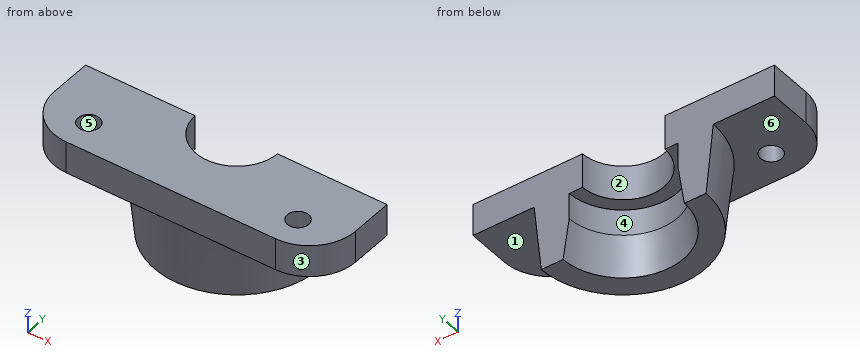
from build123d import *
from OCP.BRepAlgoAPI import BRepAlgoAPI_Cut
from OCP.TopTools import TopTools_ListOfShape

# Parameters (mm, degrees)
BOSS_EXTRUDE2_DEPTH      = 22.67949
BOSS_EXTRUDE2_DEPTH_BACK = 22.67949
SKETCH5_R                = 1.6
CUT_EXTRUDE1_DEPTH       = 29.214793281


with BuildPart() as part:
    # Sketch3 → Boss-Extrude2 (new, two sides: drawn at the far end of the back side and taken through both)
    with BuildSketch(Plane(origin=(0, 0, 0), x_dir=(0, 0, -1), z_dir=(1, 0, 0)).offset(-BOSS_EXTRUDE2_DEPTH_BACK)):
        Polygon((4.8, -13.329489609), (0, -13.329489609), (0, 0), (15, 0), (15, -12.25742641), align=None)
    extrude(amount=BOSS_EXTRUDE2_DEPTH + BOSS_EXTRUDE2_DEPTH_BACK)

    # Sketch2 → Cut-Revolve1 (revolve, cut)
    with BuildSketch(Plane(origin=(0, 0, 0), x_dir=(0, 0, -1), z_dir=(1, 0, 0))):
        Polygon((15, 0.15), (0, 0.15), (0, -6.05), (5.2, -6.05), (5.2, -8.05), (9.121020847, -8.05), (15, -8.981138823), align=None)
    revolve(axis=Axis((0, 0.15, -15), (0, 0, 1)), mode=Mode.SUBTRACT)

    # Sketch4 → Cut-Revolve2 (revolve, cut)
    with BuildSketch(Plane(origin=(0, 0.15, -14), x_dir=(0, 0, -1), z_dir=(1, 0, 0))):
        Polygon((1, 12.40742641), (-9.2, 13.479489609), (-9.2, 37.679985647), (1, 37.679985647), align=None)
    revolve(axis=Axis((0, 0.15, -14), (0, 0, 1)), mode=Mode.SUBTRACT)


with BuildPart() as cut_extrude1_tool:
    # Sketch5 → Cut-Extrude1 (new, through all)
    with BuildSketch(Plane(origin=(0, 0, -4.8), x_dir=(-1, 0, 0), z_dir=(0, 0, -1))):
        with Locations(Location((-15.748733562, -8.729489609, 0), (0, 0, 90))):
            Circle(SKETCH5_R)
        with Locations(Location((15.748733562, -8.729489609, 0), (0, 0, 270))):
            Circle(SKETCH5_R)
        with BuildLine():
            Line((-22.679489609, -13.329489609), (-22.679489609, -6.398733562))
            ThreePointArc((-22.679489609, -6.398733562), (-20.649518162, -11.299518162), (-15.748733562, -13.329489609))
            Line((-15.748733562, -13.329489609), (-22.679489609, -13.329489609))
        make_face()
        with BuildLine():
            Line((22.679489609, -13.329489609), (22.679489609, -6.398733562))
            ThreePointArc((22.679489609, -6.398733562), (20.649518162, -11.299518162), (15.748733562, -13.329489609))
            Line((15.748733562, -13.329489609), (22.679489609, -13.329489609))
        make_face()
    extrude(amount=-CUT_EXTRUDE1_DEPTH)


with BuildPart() as part_1:
    add(part.part)

    # Cut-Extrude1: cut by cut_extrude1_tool, with a tolerance
    cut_extrude1_stock = TopTools_ListOfShape()
    cut_extrude1_stock.Append(part_1.part.wrapped)
    cut_extrude1_tools = TopTools_ListOfShape()
    cut_extrude1_tools.Append(cut_extrude1_tool.part.wrapped)
    cut_extrude1_cut = BRepAlgoAPI_Cut()
    cut_extrude1_cut.SetArguments(cut_extrude1_stock)
    cut_extrude1_cut.SetTools(cut_extrude1_tools)
    cut_extrude1_cut.SetFuzzyValue(0.00001)
    cut_extrude1_cut.Build()
    add(Compound.cast(cut_extrude1_cut.Shape()).solids(), mode=Mode.REPLACE)


solid = part_1.part
For this review, take the finished solid that the model builds, in its own axes (mm). Face numbers are marked on the shaded views. A direction names the side the tool comes from. Round coordinates to 2 decimals unless told otherwise and drop trailing zeros. Order: outer loops, then holes, each group sorted by start corner. A loop starts at its lowest first (then second) coordinate and runs counter-clockwise, first axis right, second up. Notation, with made-up numbers: M 42,15.5 L 84,15.5 A17 ccw 84,39.5 Z; hole C 71.5,68.5 d11. An arc over 180 degrees is marked long. Use a Markdown table: item, result. Add a question column.
Item 1: Insertion check: pin 1 (5 mm diameter, centred on y = -6, z = -6, fed in from -X); pin 2 (4 mm diameter, centred on x = 15.5, y = -9, fed in from -Z); pin 3 (2 mm diameter, centred on y = -10.5, z = -11.5, fed in from +X); pin 4 (3 mm diameter, centred on y = -11.5, z = -12, fed in from -X). Each pin has a flat end and moves straight along its axis. Give the tip position at first contact, or say it passes through.
Item 2: Mouldability with a two-part tool opening along X and no side actions: class the marked faces 1, 2 and 3 as released by +X, released by -X, zero draft, split by the parting line, or undercut.
Item 3: Tool access review of the marked faces 4, 5 and 6: name each direction out of +Z, -Z, +X, -X, +Y, -Y from which nothing blocks a thin tool from reaching the whole face with its end or side.
Item 4: Add section D-D, the plane x = 20.5. Give the boundary of the cut face in (y, z).
Item 5: Add section B-B, the plane y = -9.75. State how many separate pieces and enclosed holes the cut face has, then the cut area to 3 significant figures.
Item 6: To check wall thickness, follow line 1 along Z through (x, y) = (9, -10.25); line 2 along X through (y, z) = (-0.75, -12); line 3 along X through (y, z) = (-2, -11.75). State the ranges of each line that lie inside material, in increasing order.
Item 7: Add section A-A, the plane z = -3. Give the boundary of the cut face in (x, y), then the cut area to 3 significant figures.
Geometry results:
| question | item | result |
|---|---|---|
| 1 | pin 1 | stops at x = -22.68 |
| 1 | pin 2 | stops at z = -4.8 |
| 1 | pin 3 | stops at x = 8.38 |
| 1 | pin 4 | stops at x = -7.69 |
| 2 | face 1 | zero draft |
| 2 | face 2 | undercut |
| 2 | face 3 | released by +X |
| 3 | face 4 | -Z, +Y |
| 3 | face 5 | +Z, -Z |
| 3 | face 6 | -Z, -X, -Y |
| 4 | outline | M -11.44,-4.8 L 0,-4.8 L 0,0 L -11.44,0 Z |
| 5 | separate pieces | 3 |
| 5 | enclosed holes | 0 |
| 5 | area | 356 mm² |
| 6 | line 1 | z = -4.8 to 0 |
| 6 | line 2 | x = -12.69 to -8.61, 8.61 to 12.69 |
| 6 | line 3 | x = -12.57 to -8.34, 8.34 to 12.57 |
| 7 | outline | M -22.68,-6.4 A6.93 ccw -15.75,-13.33 L 15.75,-13.33 A6.93 ccw 22.68,-6.4 L 22.68,0 L 6.2,0 A6.2 cw -6.2,0 L -22.68,0 Z; hole C -15.75,-8.73 d3.2; hole C 15.75,-8.73 d3.2 |
| 7 | area | 509 mm² |
